from build123d import *

# Parameters (mm, degrees)
SKETCH_1_R      = 1.65
EXTRUDE_1_DEPTH = 3
FILLET_1_R      = 10
FILLET_2_R      = 5


with BuildPart() as part:
    # 草图1 → 凸台-拉伸1 (new body)
    with BuildSketch(Plane.XY):
        Polygon((-14.5, -5), (14.5, -5), (14.5, 35), (-109.652000503, 80.187632708), (-174.042829775, 172.147267185), (-197.798239059, 155.513550531), (-128.162819072, 56.063864277), (-14.5, 14.693981392), align=None)
        Circle(SKETCH_1_R, mode=Mode.SUBTRACT)
        with Locations((0, 30)):
            Circle(SKETCH_1_R, mode=Mode.SUBTRACT)
        with Locations((-183.052652235, 159.734648636)):
            Circle(SKETCH_1_R, mode=Mode.SUBTRACT)
        with Locations((-165.845359145, 135.160087308)):
            Circle(SKETCH_1_R, mode=Mode.SUBTRACT)
        with Locations((-148.638066054, 110.585525979)):
            Circle(SKETCH_1_R, mode=Mode.SUBTRACT)
        with Locations((-131.430772964, 86.01096465)):
            Circle(SKETCH_1_R, mode=Mode.SUBTRACT)
    extrude(amount=EXTRUDE_1_DEPTH)

    # 圆角1
    fillet_1_edges = [part.edges().sort_by_distance(p)[0] for p in [
        (-14.5, 14.693981392, 1.5),
        (-128.162819072, 56.063864277, 1.5),
        (-109.652000503, 80.187632708, 1.5),
        (14.5, 35, 1.5),
    ]]
    fillet(fillet_1_edges, radius=FILLET_1_R)

    # 圆角2
    fillet_2_edges = [part.edges().sort_by_distance(p)[0] for p in [
        (-197.798239059, 155.513550531, 1.5),
        (-174.042829775, 172.147267185, 1.5),
        (14.5, -5, 1.5),
        (-14.5, -5, 1.5),
    ]]
    fillet(fillet_2_edges, radius=FILLET_2_R)


solid = part.part
The model under review builds one solid part; all positions refer to its coordinate system, in mm. Coordinates: 2 decimals unless noted, no trailing zeros. Write each loop counter-clockwise with the first axis right and the second up, starting at its lowest first coordinate (ties: lowest second). Pieces come first, ordered by that corner, then holes. Notation, with made-up numbers: (-19, 48.5) - (-2, 48.5) arc R30 cw to (-2, 74.5) - close; hole circle Ø9 at (32, -7.75). An arc over 180 degrees is marked (long way). Answer as a JSON object with one key per item and string values. Group by question number.
1. To check wall thickness, follow probe 1 along Y at (x, z) = (0, 1); probe 2 along X at (y, z) = (6, 0.4); probe 3 along X at (y, z) = (136, 1.35). State the ranges of each line that lie inside material, in increasing order.
2. Add section A-A (z = 1.3). Give the boundary of the cut face in (x, y).
3. Clearance check with flat-ended pins moving along their axes: pin 1 Ø2 at (x, y) = (-165.85, 135.16) entering from -Z; pin 2 Ø1.5 at (y, z) = (2, 1.5) entering from -X. State where each tip first meets the part, or that it passes through.
4. Add section B-B (y = 155.5). Give the boundary of the cut face in (x, z).
5. Add section C-C (x = -6.5). Give the boundary of the cut face in (y, z).
Findings:
{
 "1": {"probe 1": "-5 to -1.65, 1.65 to 28.35, 31.65 to 40.28", "probe 2": "-14.5 to 14.5", "probe 3": "-184.13 to -167.27, -164.43 to -148.73"},
 "2": {"outline": "(-194.93, 151.42) - (-129.97, 58.65) arc R10 ccw to (-125.2, 54.99) - (-21.08, 17.09) arc R10 cw to (-14.5, 7.69) - (-14.5, 0) arc R5 ccw to (-9.5, -5) - (9.5, -5) arc R5 ccw to (14.5, 0) - (14.5, 28) arc R10 ccw to (7.92, 37.39) - (-106.69, 79.11) arc R10 cw to (-111.46, 82.77) - (-171.17, 168.05) arc R5 ccw to (-178.14, 169.28) - (-193.7, 158.38) arc R5 ccw to start; hole circle Ø3.3 at (-183.05, 159.73); hole circle Ø3.3 at (-165.85, 135.16); hole circle Ø3.3 at (-148.64, 110.59); hole circle Ø3.3 at (-131.43, 86.01); hole circle Ø3.3 at (0, 0); hole circle Ø3.3 at (0, 30)"},
 "3": {"pin 1": "through", "pin 2": "x = -14.5"},
 "4": {"outline": "(-195.68, 0) - (-162.39, 0) - (-162.39, 3) - (-195.68, 3) - close"},
 "5": {"outline": "(-5, 0) - (42.64, 0) - (42.64, 3) - (-5, 3) - close"}
}
